```python
from build123d import *

# Parameters (mm, degrees)
REVOLVE1_ANGLE     = 180
CUT_EXTRUDE3_DEPTH = 50
SKETCH4_R          = 2
CUT_EXTRUDE4_DEPTH = 43


with BuildPart() as part:
    # Sketch1 → Revolve1 (revolve)
    with BuildSketch(Plane.XY):
        Polygon((25, 0), (-25, 0), (-25, 25), (-18, 25), (-18, 19), (-11, 19), (-11, 17.5), (11, 17.5), (11, 19), (18, 19), (18, 25), (25, 25), align=None)
    revolve(axis=Axis((-38.949360705, 0, 0), (1, 0, 0)), revolution_arc=REVOLVE1_ANGLE)

    # Sketch2 → Cut-Extrude3 (cut)
    with BuildSketch(Plane.ZY.offset(25)):
        with BuildLine():
            Line((0, 12.5), (0, -12.5))
            ThreePointArc((0, -12.5), (12.5, 0), (0, 12.5))
        make_face()
    extrude(amount=-CUT_EXTRUDE3_DEPTH, mode=Mode.SUBTRACT)

    # Sketch4 → Cut-Extrude4 (cut)
    with BuildSketch(Plane(origin=(0, 0, 17.5), x_dir=(-1, 0, 0), z_dir=(0, 0, -1))):
        Circle(SKETCH4_R)
    extrude(amount=CUT_EXTRUDE4_DEPTH, mode=Mode.SUBTRACT)


solid = part.part
```
Here's how the part is built. I have some questions about the finished solid (model axes, mm). A direction names the side the tool comes from. Coordinates: 2 decimals unless noted, no trailing zeros. Write each loop counter-clockwise with the first axis right and the second up, starting at its lowest first coordinate (ties: lowest second). Pieces come first, ordered by that corner, then holes. Notation, with made-up numbers: (89, 43.5) - (126, 43.5) arc R22 ccw to (126, 78.5) - close; hole circle Ø8 at (20.5, 62.25). An arc over 180 degrees is marked (long way). One line per item, written item: value.
1) I need wall thicknesses on line 1 along X through (y, z) = (0, 13.6); line 2 along X through (y, z) = (-8, 19.5); line 3 along Y through (x, z) = (0, 13.7). Which ranges of each line are inside material? Lowest first, please.
Model answer:
line 1: x = -25 to -2, 2 to 25
line 2: x = -25 to -18, 18 to 25
line 3: y = -10.89 to -2, 2 to 10.89
2) Suppose I cut it at D-D on z = 14. Write out the boundary of the cut face in (x, y).
Model answer:
outline: (-25, -20.71) - (-18, -20.71) - (-18, -12.85) - (-11, -12.85) - (-11, -10.5) - (11, -10.5) - (11, -12.85) - (18, -12.85) - (18, -20.71) - (25, -20.71) - (25, 20.71) - (18, 20.71) - (18, 12.85) - (11, 12.85) - (11, 10.5) - (-11, 10.5) - (-11, 12.85) - (-18, 12.85) - (-18, 20.71) - (-25, 20.71) - close; hole circle Ø4 at (0, 0)
3) I'm going to push flat-ended pins straight in: P1, Ø10, axis at x = 17, y = -0.5, coming from the -Z side (3 decimals); P2, Ø3, axis at x = -3, y = -8.5, coming from the -Z side; P3, Ø1.5, axis at x = -14.5, y = -3, coming from the -Z side. Where does each tip first touch, or does it pass through?
Model answer:
P1: stops at z = 11.225
P2: stops at z = 7.5
P3: stops at z = 11.92
4) We'd pull the mould along X, two halves only. Please class faces 3 (the flat face through (-25, 0, 13)), 4 (the cylindrical face through (21.549, 0.55, 24.994)), 5 (the flat face through (-18, -2, 20)): pulls with the +X half, pulls with the -X half, needs draft (parallel to the pull), parting line crosses it, or undercut.
Model answer:
face 3: pulls with the -X half
face 4: needs draft
face 5: undercut
5) Suppose I cut it at C-C on y = -6.5. Write out the boundary of the cut face in (x, z).
Model answer:
outline: (-25, 10.68) - (25, 10.68) - (25, 24.14) - (18, 24.14) - (18, 17.85) - (11, 17.85) - (11, 16.25) - (-11, 16.25) - (-11, 17.85) - (-18, 17.85) - (-18, 24.14) - (-25, 24.14) - close
6) On a 3-axis mill with a long thin cutter (end or side, diameter ignored), from which of +Z, -Z, +X, -X, +Y, -Y can I reach the whole of each face in a straight line? I mean faces 1 (the cylindrical face through (2.598, 0.385, 17.496)), 2 (the flat face through (0, -17, 0)). Say none if no direction works.
Model answer:
face 1: +Z
face 2: -Z, +X, -X, +Y, -Y
7) Suppose I cut it at B-B on x = 0. Write out the boundary of the cut face in (y, z), and give its area (3 significant figures).
Model answer:
outline: (-17.5, 0) - (-12.5, 0) arc R12.5 cw to (-2, 12.34) - (-2, 17.39) arc R17.5 ccw to start; (2, 12.34) arc R12.5 cw to (12.5, 0) - (17.5, 0) arc R17.5 ccw to (2, 17.39) - close
area: 216 mm²
8) Suppose I cut it at A-A on z = 10.25. Write out the boundary of the cut face in (x, y).
Model answer:
outline: (-25, -22.8) - (-18, -22.8) - (-18, -16) - (-11, -16) - (-11, -14.18) - (11, -14.18) - (11, -16) - (18, -16) - (18, -22.8) - (25, -22.8) - (25, -7.15) - (-25, -7.15) - close; (-25, 7.15) - (25, 7.15) - (25, 22.8) - (18, 22.8) - (18, 16) - (11, 16) - (11, 14.18) - (-11, 14.18) - (-11, 16) - (-18, 16) - (-18, 22.8) - (-25, 22.8) - close
